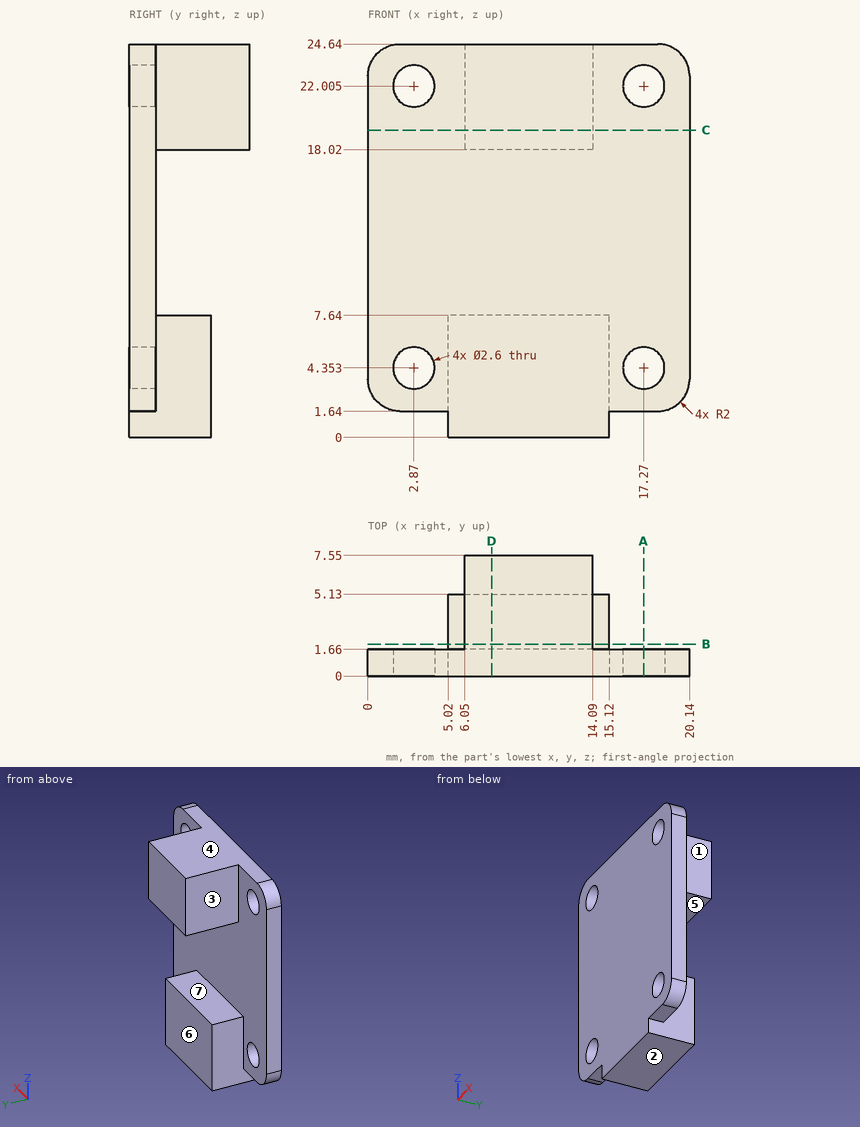
Could you check a few things on this drawing? It's one solid part, dimensions in mm from its lowest x, y, z. A direction names the side the tool comes from. Round coordinates to 2 decimals unless told otherwise and drop trailing zeros. Order: outer loops, then holes, each group sorted by start corner. A loop starts at its lowest first (then second) coordinate and runs counter-clockwise, first axis right, second up. Notation, with made-up numbers: (-25, 10.25) -> (21, 10.25) arc R38 cw to (21, 49.25) -> close; hole circle Ø10 at (-4, -31). An arc over 180 degrees is marked (long way). One line per question, with ' | ' between items.
Q1. If I drill on line 1 (Z direction, x = 17.27, y = 0.85) (1 decimal); line 2 (Z direction, x = 12.5, y = 5); line 3 (Y direction, x = 14.75, z = 17.25), over which ranges is the centre line in solid material (lowest first)? Write a range as from..to.
Computed values:
line 1: 1.6..3.1, 5.7..20.7, 23.3..24.6 | line 2: 0..7.64, 18.02..24.64 | line 3: 0..1.66
Q2. I'm going to push flat-ended pins straight in: pin 1 (6 mm diameter, centred on x = 7.5, z = 17, fed in from +Y); pin 2 (1.8 mm diameter, centred on y = 4, z = 23, fed in from +X); pin 3 (1.3 mm diameter, centred on x = 3.5, y = 1, fed in from -Z); pin 4 (1.6 mm diameter, centred on x = 17.27, z = 22.01, fed in from +Y). Where does each tip first touch, or does it pass through?
Computed values:
pin 1: y = 7.55 | pin 2: x = 14.09 | pin 3: z = 1.64 | pin 4: through
Q3. If we section it at A-A on x = 17.27: Write out the boundary of the cut face in (y, z) (1 decimal).
Computed values:
outline: (0, 1.6) -> (1.7, 1.6) -> (1.7, 3.1) -> (0, 3.1) -> close; (0, 5.7) -> (1.7, 5.7) -> (1.7, 20.7) -> (0, 20.7) -> close; (0, 23.3) -> (1.7, 23.3) -> (1.7, 24.6) -> (0, 24.6) -> close
Q4. If we section it at C-C on z = 19.25: Write out the boundary of the cut face in (x, y).
Computed values:
outline: (0, 0) -> (20.14, 0) -> (20.14, 1.66) -> (14.09, 1.66) -> (14.09, 7.55) -> (6.05, 7.55) -> (6.05, 1.66) -> (0, 1.66) -> close
Q5. Which directions (+Z, -Z, +X, -X, +Y, -Y) give clear straight access to the entire face, cutting with the end or side of a thin tool? Please do the marked faces 1, 2 and 3.
Computed values:
face 1: +Z, +X, +Y | face 2: -Z, +X, -X, +Y, -Y | face 3: +Z, -X, +Y
Q6. If we section it at B-B on y = 2: Write out the boundary of the cut face in (x, z).
Computed values:
outline: (5.02, 0) -> (15.12, 0) -> (15.12, 7.64) -> (5.02, 7.64) -> close; (6.05, 18.02) -> (14.09, 18.02) -> (14.09, 24.64) -> (6.05, 24.64) -> close
Q7. If we section it at D-D on x = 7.75: Write out the boundary of the cut face in (y, z), plus the area to 3 significant figures.
Computed values:
outline: (0, 0) -> (5.13, 0) -> (5.13, 7.64) -> (1.66, 7.64) -> (1.66, 18.02) -> (7.55, 18.02) -> (7.55, 24.64) -> (0, 24.64) -> close | area: 106 mm²
Q8. We'd pull the mould along Z, two halves only. Please class the marked faces 4, 5, 6 and 7: released by +Z, released by -Z, zero draft, split by the parting line, or undercut.
Computed values:
face 4: released by +Z | face 5: undercut | face 6: zero draft | face 7: undercut
